Geometry: see drawing. Coordinates: mm, zero at the bounding-box minimum. Give positions to 0.01 mm unless a question says otherwise; leave off trailing zeros. Write each loop counter-clockwise with the first axis right and the second up, starting at its lowest first coordinate (ties: lowest second). Pieces come first, ordered by that corner, then holes. Notation, with made-up numbers: M -9.5,78 L 10.5,78 A21 cw 10.5,111 Z; hole C 50,-32 d1. An arc over 180 degrees is marked long. Use a Markdown table: item, result. Add a question column.
1) Section A-A on y = 5. Return the cut outline in (x, z), then the cut area to 3 significant figures.
2) Pin query (flat end, axial travel): pin 1 (1 mm diameter, centred on x = 33.5, z = 1.5, fed in from -Y). Return the tip coordinate at first contact, or that it passes through.
3) Line query: line 1 (Y direction, x = 5, z = 1.4); line 2 (X direction, y = 5, z = 1.3); line 3 (X direction, y = 145, z = 1.05). Output: solid intervals per line, ascending.
4) Section C-C on y = 145. Return the cut outline in (x, z).
5) Section B-B on x = 5. Return the cut outline in (y, z).
6) Section D-D on z = 0.45. Return the cut outline in (x, y).
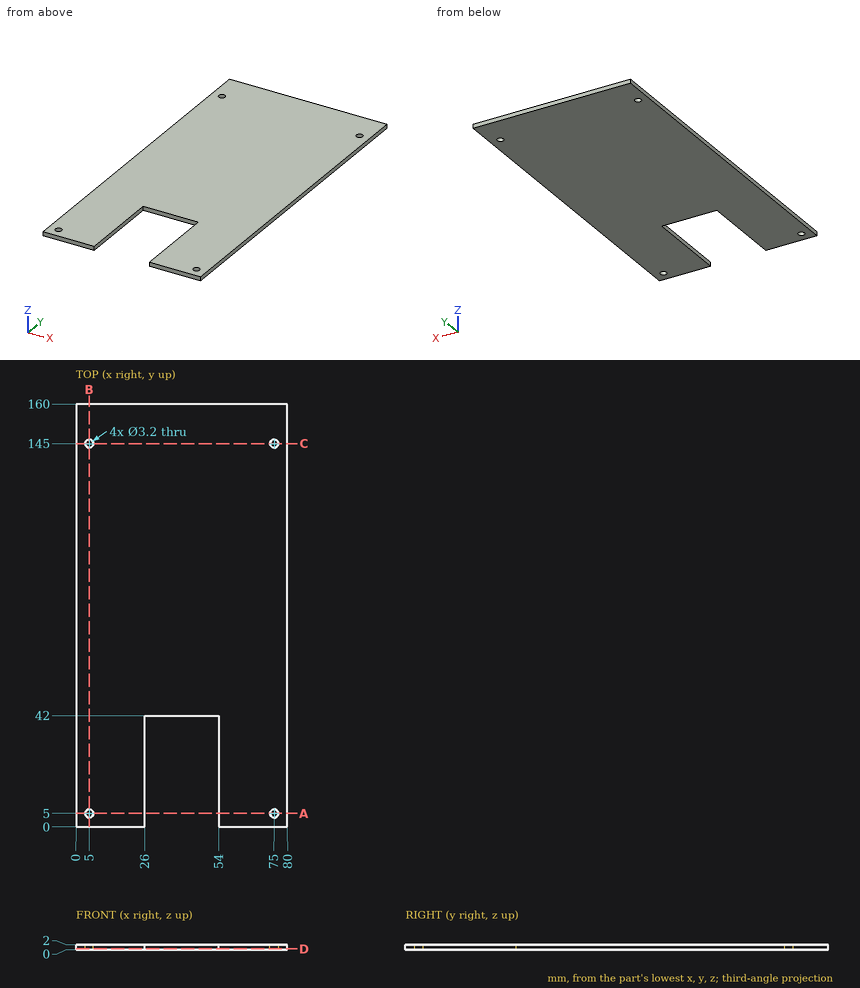
Found:
| question | item | result |
|---|---|---|
| 1 | outline | M 0,0 L 3.4,0 L 3.4,2 L 0,2 Z; M 6.6,0 L 26,0 L 26,2 L 6.6,2 Z; M 54,0 L 73.4,0 L 73.4,2 L 54,2 Z; M 76.6,0 L 80,0 L 80,2 L 76.6,2 Z |
| 1 | area | 91.2 mm² |
| 2 | pin 1 | y = 42 |
| 3 | line 1 | 0 to 3.4, 6.6 to 143.4, 146.6 to 160 |
| 3 | line 2 | 0 to 3.4, 6.6 to 26, 54 to 73.4, 76.6 to 80 |
| 3 | line 3 | 0 to 3.4, 6.6 to 73.4, 76.6 to 80 |
| 4 | outline | M 0,0 L 3.4,0 L 3.4,2 L 0,2 Z; M 6.6,0 L 73.4,0 L 73.4,2 L 6.6,2 Z; M 76.6,0 L 80,0 L 80,2 L 76.6,2 Z |
| 5 | outline | M 0,0 L 3.4,0 L 3.4,2 L 0,2 Z; M 6.6,0 L 143.4,0 L 143.4,2 L 6.6,2 Z; M 146.6,0 L 160,0 L 160,2 L 146.6,2 Z |
| 6 | outline | M 0,0 L 26,0 L 26,42 L 54,42 L 54,0 L 80,0 L 80,160 L 0,160 Z; hole C 5,5 d3.2; hole C 5,145 d3.2; hole C 75,5 d3.2; hole C 75,145 d3.2 |
